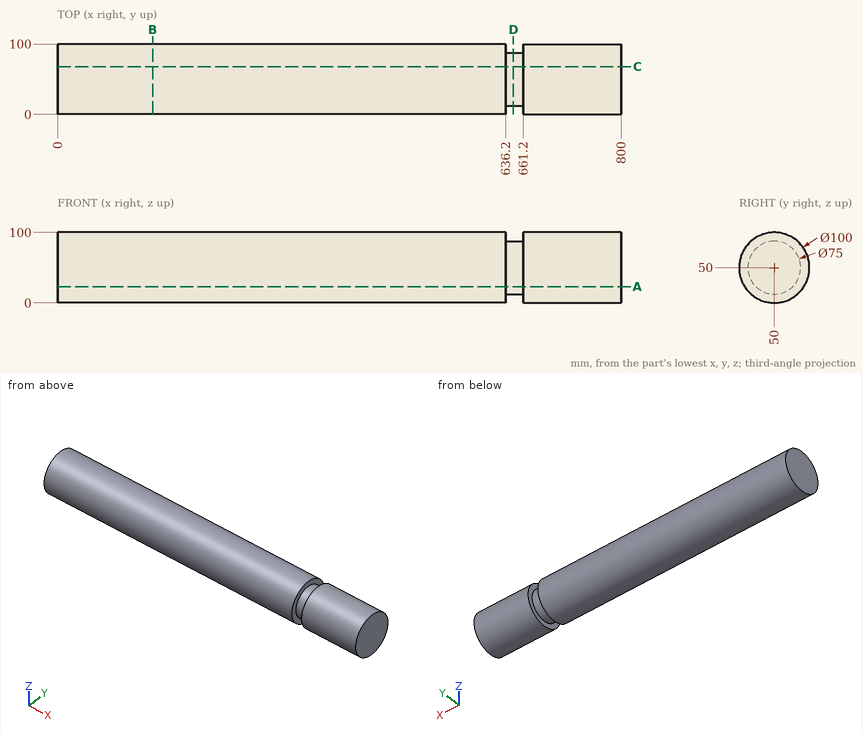
The figure shows three views and two pictorial views of one solid part (mm, origin at its lowest corner). Answer the questions. Coordinates: 2 decimals unless noted, no trailing zeros. Loops run counter-clockwise (first coordinate to the right, second up) from the corner with the lowest first, then second, coordinate; pieces in that order, holes last. Notation, with made-up numbers: (50, 61) - (100, 61) arc R34 cw to (100, 98) - close; hole circle Ø4 at (73, 81). An arc over 180 degrees is marked (long way). Use a Markdown table: item, result. Add a question column.
1) The part is cut by section D-D, the plane x = 647. Give the vertices of the cut face in (y, z), and give its area (3 significant figures).
2) The part is cut by section A-A, the plane z = 23. Give the vertices of the cut face in (x, y).
3) The part is cut by section B-B, the plane x = 135. Give the vertices of the cut face in (y, z), and give its area (3 significant figures).
4) Find the intervals of material crossed by line 1 (X direction, y = 16, z = 33.5); line 2 (Z direction, x = 556.5, y = 53); line 3 (Y direction, x = 410, z = 14.5), in increasing order.
5) The part is cut by section C-C, the plane y = 68. Give the vertices of the cut face in (x, z).
6) Given pin 1 (4 mm diameter, centred on x = 145, y = 67.5, fed in from +Z); pin 2 (12 mm diameter, centred on x = 384.5, y = 45, fed in from -Z); pin 3 (12 mm diameter, centred on x = 323.5, z = 30.5, fed in from -Y); pin 4 (1 mm diameter, centred on x = 685, z = 37, fed in from +Y), each flat-ended and moving along its own axis, determine where each tip first touches the part or whether it passes through.
Here are the results:
| question | item | result |
|---|---|---|
| 1 | outline | circle Ø75 at (50, 50) |
| 1 | area | 4,420 mm^2 |
| 2 | outline | (0, 7.92) - (636.2, 7.92) - (636.2, 23.98) - (661.2, 23.98) - (661.2, 7.92) - (800, 7.92) - (800, 92.08) - (661.2, 92.08) - (661.2, 76.02) - (636.2, 76.02) - (636.2, 92.08) - (0, 92.08) - close |
| 3 | outline | circle Ø100 at (50, 50) |
| 3 | area | 7,850 mm^2 |
| 4 | line 1 | x = 0 to 636.2, 661.2 to 800 |
| 4 | line 2 | z = 0.09 to 99.91 |
| 4 | line 3 | y = 14.79 to 85.21 |
| 5 | outline | (0, 3.35) - (636.2, 3.35) - (636.2, 17.1) - (661.2, 17.1) - (661.2, 3.35) - (800, 3.35) - (800, 96.65) - (661.2, 96.65) - (661.2, 82.9) - (636.2, 82.9) - (636.2, 96.65) - (0, 96.65) - close |
| 6 | pin 1 | stops at z = 97.54 |
| 6 | pin 2 | stops at z = 0 |
| 6 | pin 3 | stops at y = 1.86 |
| 6 | pin 4 | stops at y = 98.41 |
